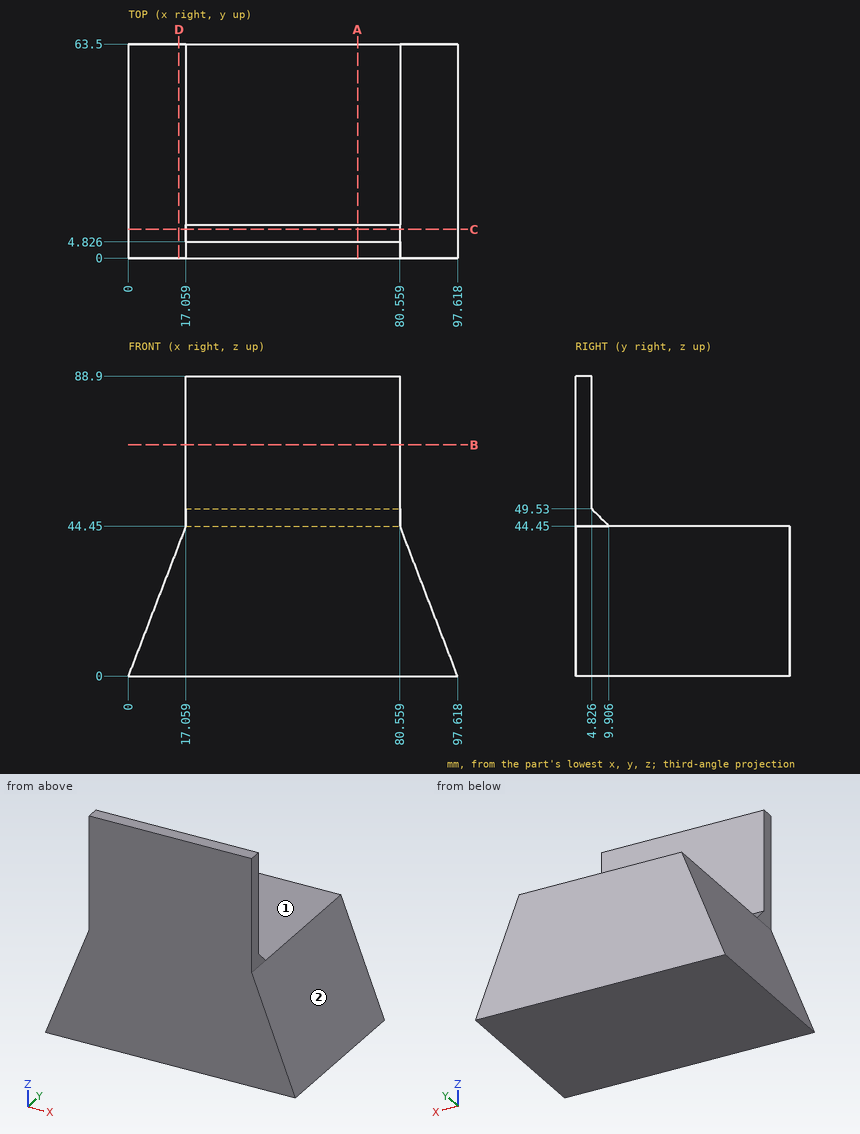
Geometry: see drawing. Coordinates: mm, zero at the bounding-box minimum. A direction names the side the tool comes from. Give positions to 0.01 mm unless a question says otherwise; leave off trailing zeros. Write each loop counter-clockwise with the first axis right and the second up, starting at its lowest first coordinate (ties: lowest second). Pieces come first, ordered by that corner, then holes. Notation, with made-up numbers: (54.25, -7.75) -> (80.25, -7.75) arc R25 ccw to (80.25, 29.25) -> close; hole circle Ø5 at (61, 82.25). An arc over 180 degrees is marked (long way). Use one line per item in the form item = value. Start each with the question number.
1) Section query A-A on x = 68. Return the cut outline in (y, z).
2) Section query B-B on z = 68.5. Return the cut outline in (x, y).
3) Section query D-D on x = 15. Return the cut outline in (y, z) (1 decimal).
4) Pin query (flat end, axial travel): pin 1 (5 mm diameter, centred on y = 5, z = 71, fed in from +X); pin 2 (2 mm diameter, centred on x = 68, z = 67.5, fed in from +Y); pin 3 (2 mm diameter, centred on y = 9, z = 26, fed in from -X) (1 decimal); pin 4 (1.5 mm diameter, centred on x = 77.5, y = 32.5, fed in from -Z). Return the tip coordinate at first contact, or that it passes through.
5) Ray query, probe 1 along Z at (x, y) = (67, 32.5); probe 2 along Y at (x, z) = (79, 77); probe 3 along X at (y, z) = (45, 12) (1 decimal). Return the intervals inside material, ascending. Write a range as from..to.
6) Set-up query: the marked faces 1 and 2. Return all of +Z, -Z, +X, -X, +Y, -Y with unobstructed straight access to the full face (end or side cutting, diameter ignored); none if empty.
7) Section query C-C on y = 8.5. Return the cut outline in (x, z), then the cut area to 3 significant figures.
Outcome:
q1.outline = (0, 0) -> (63.5, 0) -> (63.5, 44.45) -> (9.91, 44.45) -> (4.83, 49.53) -> (4.83, 88.9) -> (0, 88.9) -> close
q2.outline = (17.06, 0) -> (80.56, 0) -> (80.56, 4.83) -> (17.06, 4.83) -> close
q3.outline = (0, 0) -> (63.5, 0) -> (63.5, 39.1) -> (0, 39.1) -> close
q4.pin_1 = 80.56
q4.pin_2 = 4.83
q4.pin_3 = 9.6
q4.pin_4 = 0
q5.probe_1 = 0..44.45
q5.probe_2 = 0..4.83
q5.probe_3 = 4.6..93
q6.face_1 = +Z, +X, -X, +Y
q6.face_2 = +Z, +X, +Y, -Y
q7.outline = (0, 0) -> (97.62, 0) -> (80.56, 44.45) -> (80.56, 45.86) -> (17.06, 45.86) -> (17.06, 44.45) -> close
q7.area = 3,670 mm^2
